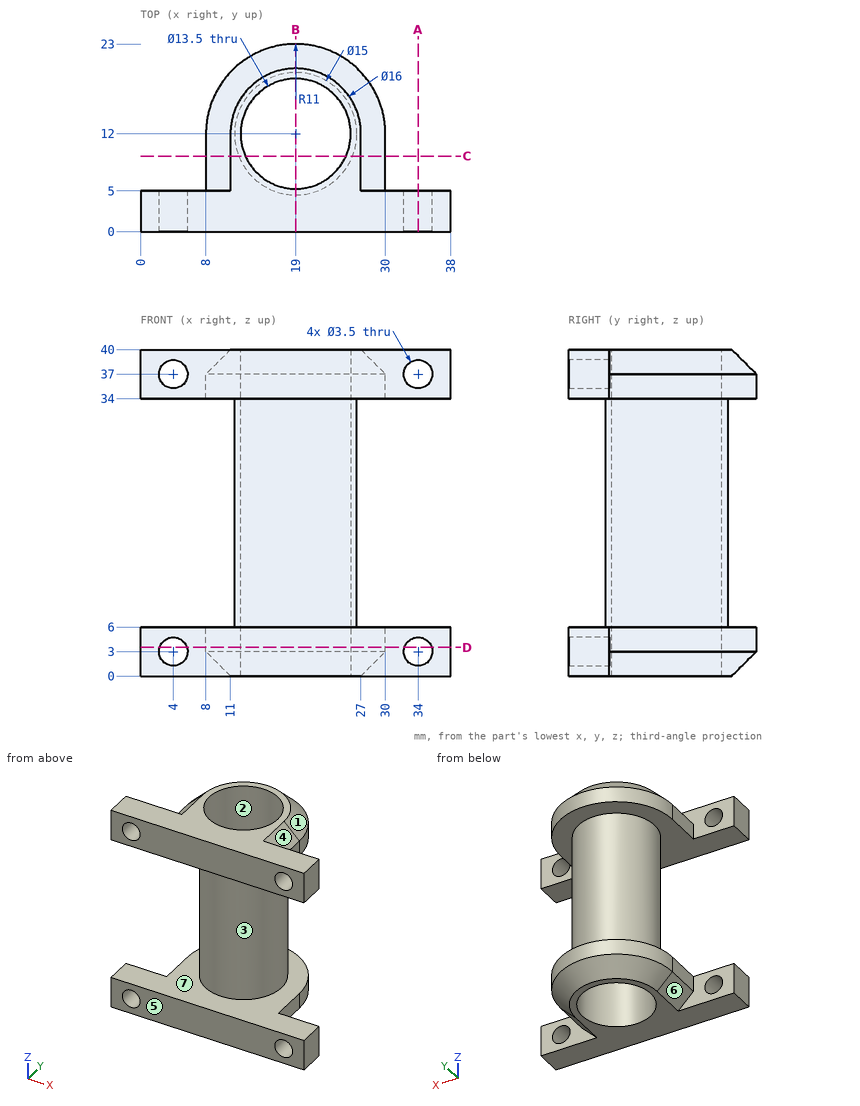
Here's the drawing with two shaded views (mm, measured from the low corner). I have some questions. A direction names the side the tool comes from. Give positions to 0.01 mm unless a question says otherwise; leave off trailing zeros. Order: outer loops, then holes, each group sorted by start corner. A loop starts at its lowest first (then second) coordinate and runs counter-clockwise, first axis right, second up. Notation, with made-up numbers: (37, 79) -> (91, 79) arc R22 ccw to (91, 110) -> close; hole circle Ø2 at (45.5, 88). An arc over 180 degrees is marked (long way). One line per item, written item: value. Start each with the question number.
1. I need wall thicknesses on probe 1 along X at (y, z) = (1.8, 37); probe 2 along Z at (x, y) = (24, 3); probe 3 along Y at (x, z) = (19, 30.5). Which ranges of each line are inside material? Lowest first, please. Write a range as from..to.
2. For the marked faces 4, 5, 6 and 7, which set-ups out of +Z, -Z, +X, -X, +Y, -Y let a thin tool reach every point of the face, with its end or its side?
3. Imagine slicing it at B-B, the plane x = 19. List the corners of the cut face in (y, z) for me, plus the area to 3 significant figures.
4. Imagine slicing it at D-D, the plane z = 3.5. List the corners of the cut face in (x, y) for me, plus the area to 3 significant figures.
5. We'd pull the mould along Z, two halves only. Please class the marked faces 1, 2 and 3: released by +Z, released by -Z, zero draft, split by the parting line, or undercut.
6. Imagine slicing it at A-A, the plane x = 34. List the corners of the cut face in (y, z) for me.
7. Imagine slicing it at C-C, the plane y = 9.25. List the corners of the cut face in (x, z) for me.
8. Will these pins go through, and if not, where does the flat tip stop? pin 1 Ø3 at (x, z) = (34.5, 2.5) entering from +Y; pin 2 Ø0.9 at (y, z) = (8, 4.5) entering from -X; pin 3 Ø3.5 at (y, z) = (7, 36) entering from +X.
Values follow:
1. probe 1: x = 0..2.25, 5.75..32.25, 35.75..38
1. probe 2: z = 0..6, 34..40
1. probe 3: y = 4.5..5.25, 18.75..19.5
2. face 4: +Z, +X, +Y
2. face 5: +Z, -Z, +X, -X, -Y
2. face 6: -Z, -X, +Y
2. face 7: none
3. outline: (0, 0) -> (5.25, 0) -> (5.25, 40) -> (0, 40) -> (0, 34) -> (4.5, 34) -> (4.5, 6) -> (0, 6) -> close; (18.75, 0) -> (20, 0) -> (23, 3) -> (23, 6) -> (19.5, 6) -> (19.5, 34) -> (23, 34) -> (23, 37) -> (20, 40) -> (18.75, 40) -> close
3. area: 147 mm2
4. outline: (0, 0) -> (2.32, 0) -> (2.32, 5) -> (0, 5) -> close; (5.68, 0) -> (32.32, 0) -> (32.32, 5) -> (30, 5) -> (30, 12) arc R11 ccw to (8, 12) -> (8, 5) -> (5.68, 5) -> close; (35.68, 0) -> (38, 0) -> (38, 5) -> (35.68, 5) -> close; hole circle Ø13.5 at (19, 12)
4. area: 357 mm2
5. face 1: released by +Z
5. face 2: zero draft
5. face 3: undercut
6. outline: (0, 0) -> (5, 0) -> (5, 1.25) -> (0, 1.25) -> close; (0, 4.75) -> (5, 4.75) -> (5, 6) -> (0, 6) -> close; (0, 34) -> (5, 34) -> (5, 35.25) -> (0, 35.25) -> close; (0, 38.75) -> (5, 38.75) -> (5, 40) -> (0, 40) -> close
7. outline: (8, 3) -> (11, 0) -> (12.84, 0) -> (12.84, 40) -> (11, 40) -> (8, 37) -> (8, 34) -> (12.02, 34) -> (12.02, 6) -> (8, 6) -> close; (25.16, 0) -> (27, 0) -> (30, 3) -> (30, 6) -> (25.98, 6) -> (25.98, 34) -> (30, 34) -> (30, 37) -> (27, 40) -> (25.16, 40) -> close
8. pin 1: stops at y = 5
8. pin 2: stops at x = 8
8. pin 3: stops at x = 30
